The figure shows three views and two pictorial views of one solid part (mm, origin at its lowest corner). Answer the questions. A direction names the side the tool comes from. Coordinates: 2 decimals unless noted, no trailing zeros. Write each loop counter-clockwise with the first axis right and the second up, starting at its lowest first coordinate (ties: lowest second). Pieces come first, ordered by that corner, then holes.
Item 1: Straight lines are drawn through the part: probe 1 along Y at (x, z) = (2.35, 9); probe 2 along Z at (x, y) = (1.25, 3.75); probe 3 along Y at (x, z) = (3.2, 4.75). For each, find the intervals that lie inside material, in ascending order.
Item 2: This flat-tipped pin is pushed along its axis until it touches: P1, Ø1.5, axis at x = 4, z = 1.5, coming from the -Y side. Where does it stop, or does it pass through?
Item 3: Section A-A (x = 2.35) is taken. Give the vertices of the cut face in (y, z), then the cut area to 3 significant figures.
Item 4: A tool of negligible diameter and unlimited length cuts with its end or side. For the marked faces 1 and 2, from which of +Z, -Z, +X, -X, +Y, -Y can it reach the whole face along a straight path? Write none if from no direction.
Item 5: Section C-C (z = 8.25) is taken. Give the vertices of the cut face in (x, y).
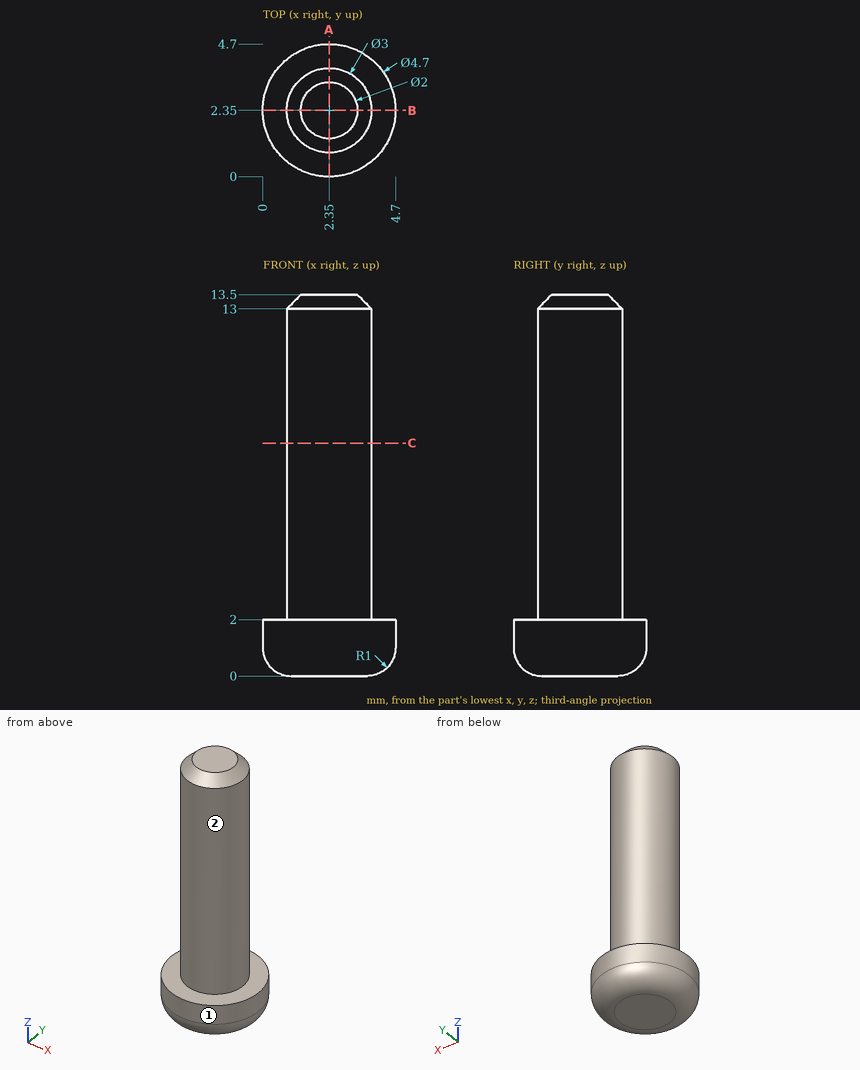
Established:
1. probe 1: y = 0.85 to 3.85
1. probe 2: z = 0.1 to 2
1. probe 3: y = 1.11 to 3.59
2. P1: stops at y = 0.18
3. outline: (0, 1) arc R1 ccw to (1, 0) - (3.7, 0) arc R1 ccw to (4.7, 1) - (4.7, 2) - (3.85, 2) - (3.85, 13) - (3.35, 13.5) - (1.35, 13.5) - (0.85, 13) - (0.85, 2) - (0, 2) - close
3. area: 43.2 mm2
4. face 1: +Z, -Z
4. face 2: +Z
5. outline: circle Ø3 at (2.35, 2.35)
